The drawing under review shows one solid part. Ordinate dimensions are in mm from its lowest x, y, z. Coordinates: 2 decimals unless noted, no trailing zeros. Order: outer loops, then holes, each group sorted by start corner. A loop starts at its lowest first (then second) coordinate and runs counter-clockwise, first axis right, second up.
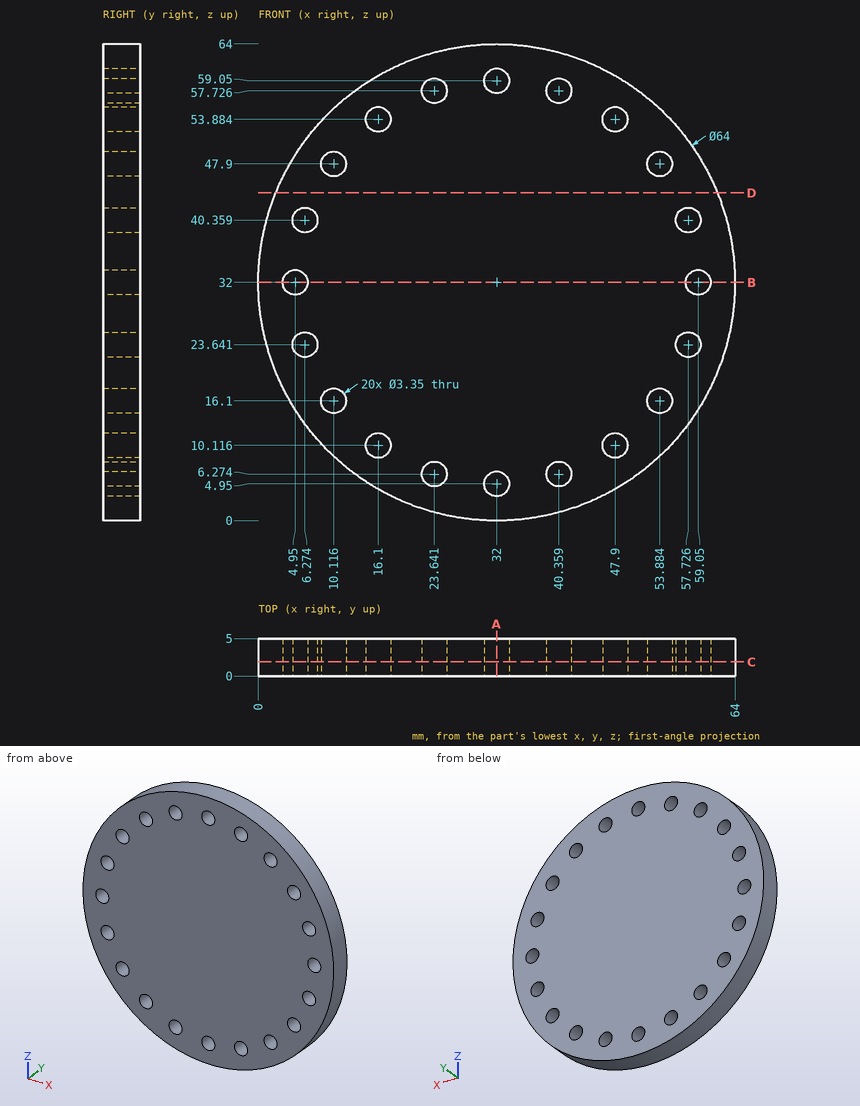
1. Clearance check with flat-ended pins moving along their axes: pin 1 Ø1 at (x, y) = (43.5, 3) entering from +Z; pin 2 Ø1.5 at (x, y) = (51, 3.5) entering from -Z (1 decimal); pin 3 Ø1 at (y, z) = (1, 7) entering from +X (1 decimal). State where each tip first meets the part, or that it passes through.
Answer below:
pin 1: stops at z = 62.05
pin 2: stops at z = 5.7
pin 3: stops at x = 52.6
2. Take a section at C-C, the plane y = 1.9. Give the number of separate pieces and of enclosed holes in the cut face, plus the area to 3 significant figures.
Answer below:
separate pieces: 1
enclosed holes: 20
area: 3,040 mm2
3. Take a section at B-B, the plane z = 32. Give the boundary of the cut face in (x, y) (1 decimal).
Answer below:
outline: (0, 0) - (3.3, 0) - (3.3, 5) - (0, 5) - close; (6.6, 0) - (57.4, 0) - (57.4, 5) - (6.6, 5) - close; (60.7, 0) - (64, 0) - (64, 5) - (60.7, 5) - close
4. Take a section at D-D, the plane z = 44. Give the boundary of the cut face in (x, y) (1 decimal), plus the area to 3 significant figures.
Answer below:
outline: (2.3, 0) - (61.7, 0) - (61.7, 5) - (2.3, 5) - close
area: 297 mm2
5. To check wall thickness, follow L1, parallel to X at y = 4.15, z = 53.5; L2, parallel to X at y = 0.8, z = 5.5 (1 decimal); L3, parallel to X at y = 3.4, z = 15 (1 decimal). State the ranges of each line that lie inside material, in increasing order.
Answer below:
L1: x = 8.3 to 14.47, 17.73 to 46.27, 49.53 to 55.7
L2: x = 14.1 to 22.2, 25.1 to 30.4, 33.6 to 38.9, 41.8 to 49.9
L3: x = 4.9 to 8.9, 11.4 to 52.6, 55.1 to 59.1
6. Take a section at A-A, the plane x = 32. Give the boundary of the cut face in (y, z) (1 decimal).
Answer below:
outline: (0, 0) - (5, 0) - (5, 3.3) - (0, 3.3) - close; (0, 6.6) - (5, 6.6) - (5, 57.4) - (0, 57.4) - close; (0, 60.7) - (5, 60.7) - (5, 64) - (0, 64) - close
